Source: CAD feature listing. Evaluate the final solid. Frame: model axes, mm. Face numbers are marked on the shaded views. A direction names the side the tool comes from. Give positions to 0.01 mm unless a question says otherwise; leave off trailing zeros. Loops run counter-clockwise (first coordinate to the right, second up) from the corner with the lowest first, then second, coordinate; pieces in that order, holes last. Notation, with made-up numbers: M 24.25,-17.5 L 79.25,-17.5 A25 ccw 79.25,17.5 Z; hole C 33,61.25 d4. An arc over 180 degrees is marked long. Answer in a Markdown table with one row per item.
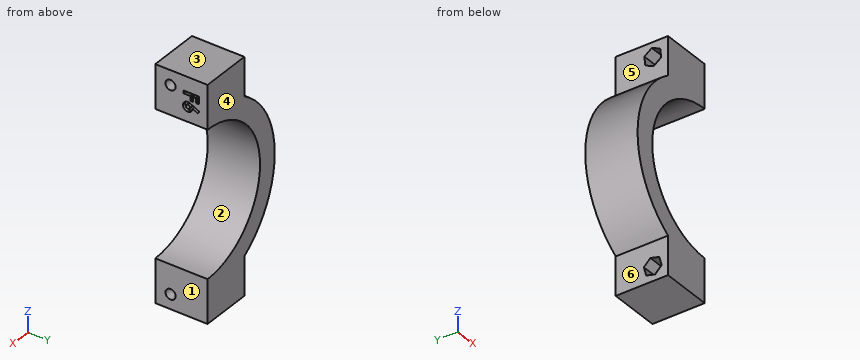
```python
from build123d import *

# Parameters (mm, degrees)
BOSS_EXTRUDE1_DEPTH = 18
SKETCH2_R           = 1.75
CUT_EXTRUDE1_DEPTH  = 33
CUT_EXTRUDE2_DEPTH  = 1
CUT_EXTRUDE3_DEPTH  = 5


with BuildPart() as part:
    # Sketch1 → Boss-Extrude1 (new body)
    with BuildSketch(Plane(origin=(0, 0, 0), x_dir=(1, 0, 0), z_dir=(0, 1, 0))):
        with BuildLine():
            Line((-11.998275301, 32.528571429), (-29.498275301, 32.528571429))
            Line((-29.498275301, 32.528571429), (-29.498275301, 19.319428078))
            ThreePointArc((-29.498275301, 19.319428078), (-21.127694429, 23.198649785), (-11.998275301, 24.528571429))
            Line((-11.998275301, 24.528571429), (-11.998275301, 32.528571429))
        make_face()
        with BuildLine():
            ThreePointArc((-11.998275301, 24.528571429), (-21.127694429, 23.198649785), (-29.498275301, 19.319428078))
            ThreePointArc((-29.498275301, 19.319428078), (-43.998275301, -7.471428571), (-29.498275301, -34.262285221))
            ThreePointArc((-29.498275301, -34.262285221), (-21.127694429, -38.141506928), (-11.998275301, -39.471428571))
            Line((-11.998275301, -39.471428571), (-11.998275301, -32.471428571))
            ThreePointArc((-11.998275301, -32.471428571), (-36.998275301, -7.471428571), (-11.998275301, 17.528571429))
            Line((-11.998275301, 17.528571429), (-11.998275301, 24.528571429))
        make_face()
        with BuildLine():
            Line((-29.498275301, -34.262285221), (-29.498275301, -47.471428571))
            Line((-29.498275301, -47.471428571), (-11.998275301, -47.471428571))
            Line((-11.998275301, -47.471428571), (-11.998275301, -39.471428571))
            ThreePointArc((-11.998275301, -39.471428571), (-21.127694429, -38.141506928), (-29.498275301, -34.262285221))
        make_face()
    extrude(amount=BOSS_EXTRUDE1_DEPTH)

    # Sketch2 → Cut-Extrude1 (cut, through all)
    with BuildSketch(Plane(origin=(-11.998275301, 0, 0), x_dir=(0, 0, -1), z_dir=(1, 0, 0))):
        with Locations((-42.471428571, 5.25)):
            Circle(SKETCH2_R)
        with Locations((27.528571429, 5.25)):
            Circle(SKETCH2_R)
    extrude(amount=-CUT_EXTRUDE1_DEPTH, mode=Mode.SUBTRACT)

    # Sketch3 → Cut-Extrude2 (cut)
    with BuildSketch(Plane(origin=(-11.998275301, 0, 0), x_dir=(0, 0, -1), z_dir=(1, 0, 0))):
        Polygon((-42.417738354, 14.960699998), (-39.839746901, 14.960699998), (-39.839746901, 14.010913673), (-41.467952029, 14.010913673), (-41.467952029, 12.993285468), (-39.839746901, 12.993285468), (-39.839746901, 12.043499143), (-41.467952029, 12.043499143), (-41.467952029, 9.669033331), (-42.417738354, 9.669033331), align=None)
        with BuildLine():
            Line((-37.418639796, 15.096383759), (-36.576976468, 14.669191918))
            Line((-36.576976468, 14.669191918), (-37.499202029, 12.857601707))
            add(Edge.make_bspline(
                [(-37.499202029, 12.857601707), (-37.444714907, 12.856212797), (-37.337743504, 12.853486031), (-37.180235064, 12.830829794), (-37.029618939, 12.792146161), (-36.884094237, 12.740675931), (-36.745768611, 12.671572146), (-36.612417045, 12.589364414), (-36.48748866, 12.48910469), (-36.368119164, 12.378021865), (-36.259577083, 12.254958161), (-36.1652891, 12.122722275), (-36.083118786, 11.984531555), (-36.01924289, 11.837294329), (-35.967718466, 11.683451224), (-35.930541327, 11.522387264), (-35.909330729, 11.353636042), (-35.906406494, 11.238995693), (-35.904917841, 11.180635228)],
                knots=[0, 0, 0, 0, 0.000163413, 0.000320819, 0.000476106, 0.000629341, 0.000782939, 0.000939124, 0.001098386, 0.001262622, 0.001427858, 0.001589654, 0.001749279, 0.001909217, 0.002070118, 0.002235459, 0.00240428, 0.002579342, 0.002579342, 0.002579342, 0.002579342], degree=3))
            add(Edge.make_bspline(
                [(-35.904917841, 11.180635228), (-35.906312832, 11.12437928), (-35.909070131, 11.013185394), (-35.931862859, 10.849869855), (-35.968697104, 10.693178147), (-36.021340637, 10.543423201), (-36.088254824, 10.399873012), (-36.170086343, 10.262611816), (-36.267513827, 10.132665321), (-36.378020019, 10.010724), (-36.498822351, 9.899573584), (-36.626154588, 9.800776626), (-36.761095728, 9.71916659), (-36.901095226, 9.650245002), (-37.048730558, 9.598814566), (-37.201792353, 9.559993497), (-37.361441325, 9.537592055), (-37.469806956, 9.534775048), (-37.524642734, 9.533349571)],
                knots=[0, 0, 0, 0, 0.000168708, 0.000333463, 0.000493643, 0.000650875, 0.000808794, 0.000968046, 0.001129383, 0.001295239, 0.001461028, 0.001621313, 0.001777843, 0.001933346, 0.002088578, 0.00224592, 0.002406475, 0.002570947, 0.002570947, 0.002570947, 0.002570947], degree=3))
            add(Edge.make_bspline(
                [(-37.524642734, 9.533349571), (-37.581984294, 9.534519384), (-37.694738713, 9.536819664), (-37.859726647, 9.562576741), (-38.017964276, 9.601350429), (-38.168562277, 9.656712667), (-38.312457177, 9.727205977), (-38.44795487, 9.814434357), (-38.576196739, 9.917435913), (-38.695815537, 10.033893272), (-38.803583159, 10.161456375), (-38.899702871, 10.293900088), (-38.981020271, 10.431432244), (-39.046844811, 10.573905795), (-39.098202644, 10.720866743), (-39.133937221, 10.872594007), (-39.157221595, 11.028685132), (-39.159951157, 11.134617402), (-39.161328098, 11.188055433)],
                knots=[0, 0, 0, 0, 0.000171885, 0.000337989, 0.000499701, 0.000660001, 0.000818339, 0.000979478, 0.001142378, 0.001311042, 0.001479484, 0.001642759, 0.00180147, 0.001957982, 0.002112862, 0.002267641, 0.002425047, 0.002585283, 0.002585283, 0.002585283, 0.002585283], degree=3))
            add(Edge.make_bspline(
                [(-39.161328098, 11.188055433), (-39.160600549, 11.229436937), (-39.159141403, 11.312430291), (-39.144477856, 11.436708329), (-39.122184114, 11.561312585), (-39.096342748, 11.666457602), (-39.06973392, 11.755368717), (-39.042951931, 11.830611792), (-39.009761556, 11.914115152), (-38.97182004, 12.006092031), (-38.927934263, 12.106431782), (-38.878333474, 12.214860904), (-38.822894189, 12.332200505), (-38.783358344, 12.412794641), (-38.76275705, 12.454790543)],
                knots=[0, 0, 0, 0, 0.000124096, 0.000248883, 0.000374888, 0.000503693, 0.000573446, 0.000653238, 0.000743197, 0.000843003, 0.000951711, 0.001071724, 0.0012007, 0.001341029, 0.001341029, 0.001341029, 0.001341029], degree=3))
            Line((-38.76275705, 12.454790543), (-37.418639796, 15.096383759))
        make_face()
        with BuildLine():
            add(Edge.make_bspline(
                [(-37.545843322, 11.975657263), (-37.59141696, 11.973566896), (-37.680598589, 11.969476324), (-37.807401527, 11.926637853), (-37.923017038, 11.859434955), (-38.023233992, 11.765841923), (-38.107056253, 11.653994574), (-38.168651791, 11.526417732), (-38.20570493, 11.384813877), (-38.209554514, 11.285806822), (-38.211541773, 11.234696726)],
                knots=[0, 0, 0, 0, 0.000136279, 0.00026668, 0.000396852, 0.0005349, 0.000675037, 0.000813949, 0.000957414, 0.001110503, 0.001110503, 0.001110503, 0.001110503], degree=3))
            add(Edge.make_bspline(
                [(-38.211541773, 11.234696726), (-38.209188797, 11.183569611), (-38.204612101, 11.084123954), (-38.166165714, 10.941171776), (-38.103217051, 10.810697813), (-38.014935565, 10.697368244), (-37.911294369, 10.603295927), (-37.796368575, 10.533724951), (-37.672075188, 10.490985217), (-37.586098416, 10.485770403), (-37.542663234, 10.483135895)],
                knots=[0, 0, 0, 0, 0.000153173, 0.000297932, 0.000440631, 0.000585017, 0.000726133, 0.000858297, 0.000985677, 0.001115733, 0.001115733, 0.001115733, 0.001115733], degree=3))
            add(Edge.make_bspline(
                [(-37.542663234, 10.483135895), (-37.496790772, 10.485817325), (-37.406826908, 10.491076074), (-37.277048133, 10.532017398), (-37.158494443, 10.600422832), (-37.053670049, 10.694193969), (-36.963627887, 10.806230295), (-36.901327806, 10.937470644), (-36.861104027, 11.081454599), (-36.856885283, 11.182470747), (-36.854704166, 11.234696726)],
                knots=[0, 0, 0, 0, 0.000137436, 0.000269537, 0.00040391, 0.000545113, 0.000689312, 0.000832011, 0.000978068, 0.001134411, 0.001134411, 0.001134411, 0.001134411], degree=3))
            add(Edge.make_bspline(
                [(-36.854704166, 11.234696726), (-36.857188856, 11.285776979), (-36.86200075, 11.384699854), (-36.898143772, 11.526967091), (-36.962674696, 11.654052204), (-37.048393503, 11.766303611), (-37.152059393, 11.85985491), (-37.272302072, 11.927167836), (-37.40489758, 11.969400428), (-37.498176409, 11.973541243), (-37.545843322, 11.975657263)],
                knots=[0, 0, 0, 0, 0.000153173, 0.000296638, 0.000436486, 0.000577899, 0.000718308, 0.000852158, 0.000988622, 0.001131234, 0.001131234, 0.001131234, 0.001131234], degree=3))
        make_face(mode=Mode.SUBTRACT)
    extrude(amount=-CUT_EXTRUDE2_DEPTH, mode=Mode.SUBTRACT)

    # Sketch4 → Cut-Extrude3 (cut)
    with BuildSketch(Plane.ZY.offset(29.498275301)):
        Polygon((-25.283205831, 3.004634402), (-24.461344982, 6.071860849), (-26.706710579, 8.317226447), (-29.773937026, 7.495365598), (-30.595797876, 4.428139151), (-28.350432278, 2.182773553), align=None)
        Polygon((44.349661379, 2.689614315), (45.627904022, 5.596404483), (43.749671214, 8.156790168), (40.593195764, 7.810385685), (39.314953121, 4.903595517), (41.193185928, 2.343209832), align=None)
    extrude(amount=-CUT_EXTRUDE3_DEPTH, mode=Mode.SUBTRACT)


solid = part.part
```
Q1. Reachability of the marked faces 4, 5 and 6 from +Z, -Z, +X, -X, +Y, -Y: full face, straight path, thin tool, end or side. Return the list, or none.
Values follow:
| item | result |
|---|---|
| face 4 | +Z, -Z, +X, -X, +Y |
| face 5 | +Z, -X, +Y, -Y |
| face 6 | -Z, -X, +Y, -Y |
Q2. Mould query, pull axis Z, two halves, no side actions, for the marked faces 1, 2 and 3. Classes: +Z half, -Z half, draft (parallel to the pull), parting line (faces both ways), or undercut.
Values follow:
| item | result |
|---|---|
| face 1 | draft |
| face 2 | undercut |
| face 3 | +Z half |
Q3. Ray query, probe 1 along X at (y, z) = (14.25, 39); probe 2 along X at (y, z) = (10.25, 33.5); probe 3 along Z at (x, y) = (-23.5, 6.5). Return the intervals inside material, ascending. Write a range as from..to.
Values follow:
| item | result |
|---|---|
| probe 1 | -29.5..-12 |
| probe 2 | -30.61..-12 |
| probe 3 | -32.53..-28.75, -26.3..-14.73, 29.67..41.25, 43.7..47.47 |
Q4. Section query A-A (x = -21.5). Output: boundary loops of the cut face in (y, z).
Values follow:
| item | result |
|---|---|
| outline | M 0,-32.53 L 18,-32.53 L 18,-15.65 L 0,-15.65 Z; M 0,30.6 L 18,30.6 L 18,47.47 L 0,47.47 Z; hole C 5.25,-27.53 d3.5; hole C 5.25,42.47 d3.5 |
Q5. Contact query for flat-ended pins moving along their axis: pin 1 Ø3 at (x, y) = (-37, 16) entering from -Z; pin 2 Ø10.5 at (y, z) = (6.5, 38.5) entering from -X; pin 3 Ø1 at (y, z) = (12, -14) entering from -X. Output: stop coordinate, or through.
Values follow:
| item | result |
|---|---|
| pin 1 | z = -14.25 |
| pin 2 | x = -30.96 |
| pin 3 | x = -36.17 |
Q6. Section query B-B (z = 23). Output: boundary loops of the cut face in (x, y).
Values follow:
| item | result |
|---|---|
| outline | M -39.98,0 L -31.59,0 L -31.59,18 L -39.98,18 Z |
Q7. Section query C-C (x = -42). Output: boundary loops of the cut face in (y, z), plus the area to 3 significant figures.
Values follow:
| item | result |
|---|---|
| outline | M 0,-3.66 L 18,-3.66 L 18,18.6 L 0,18.6 Z |
| area | 401 mm^2 |
